Part model, mm, in its own coordinate system. Face numbers are marked on the shaded views. A direction names the side the tool comes from. Give positions to 0.01 mm unless a question says otherwise; leave off trailing zeros. Loops run counter-clockwise (first coordinate to the right, second up) from the corner with the lowest first, then second, coordinate; pieces in that order, holes last. Notation, with made-up numbers: (-12.5, 56.5) -> (20.5, 56.5) arc R21 ccw to (20.5, 94.5) -> close; hole circle Ø9 at (-4, 4.5). An arc over 180 degrees is marked (long way). Write item = value, one per line.
from build123d import *

# Parameters (mm, degrees)
F0_W      = 83.106392
F0_H      = 83.106392
F1_DEPTH  = 76.2
F2_T      = -2.54
F3_W      = 78.026392
F3_H      = 78.026392
F3_W_2    = 72.946392
F3_H_2    = 72.946392
F4_DEPTH  = 2.54
F8_DEPTH  = 2.54
F9_DEPTH  = 25.4
F11_DEPTH = 2.54
F12_DEPTH = 25.4


with BuildPart() as f1:
    # F0 (on Top) → F1 (new body)
    with BuildSketch(Plane.XY):
        Rectangle(F0_W, F0_H)
    extrude(amount=F1_DEPTH)

    # F2
    f2_openings = [f1.faces().sort_by_distance(p)[0] for p in [
        (0, 0, 76.2),
    ]]
    offset(amount=F2_T, openings=f2_openings)

    # F3 (on face) → F4 (join)
    with BuildSketch(Plane(origin=(0, 0, 0), x_dir=(1, 0, 0), z_dir=(0, 0, -1))):
        Rectangle(F3_W, F3_H)
        Rectangle(F3_W_2, F3_H_2, mode=Mode.SUBTRACT)
    extrude(amount=F4_DEPTH)

    # F5 (on face) → F8 (join)
    with BuildSketch(Plane(origin=(-41.553196, 0, 0), x_dir=(0, -1, 0), z_dir=(-1, 0, 0))):
        Polygon((-23.773196, 71.12), (-36.473196, 71.12), (-36.473196, 58.42), (-31.393196, 58.42), (-31.393196, 66.04), (-23.773196, 66.04), align=None)
        Polygon((36.473196, 58.42), (36.473196, 71.12), (23.773196, 71.12), (23.773196, 66.04), (31.393196, 66.04), (31.393196, 58.42), align=None)
        Polygon((36.473196, 17.78), (31.393196, 17.78), (31.393196, 10.16), (23.773196, 10.16), (23.773196, 5.08), (36.473196, 5.08), align=None)
        Polygon((-36.473196, 17.78), (-36.473196, 5.08), (-23.773196, 5.08), (-23.773196, 10.16), (-31.393196, 10.16), (-31.393196, 17.78), align=None)
    extrude(amount=F8_DEPTH)

    # F7 (on face) → F9 (cut)
    with BuildSketch(Plane.YZ.offset(41.553196)):
        Polygon((-23.773196, 71.12), (-36.473196, 71.12), (-36.473196, 58.42), (-31.393196, 58.42), (-31.393196, 66.04), (-23.773196, 66.04), align=None)
        Polygon((36.473196, 58.42), (36.473196, 71.12), (23.773196, 71.12), (23.773196, 66.04), (31.393196, 66.04), (31.393196, 58.42), align=None)
        Polygon((23.773196, 5.08), (36.473196, 5.08), (36.473196, 17.78), (31.393196, 17.78), (31.393196, 10.16), (23.773196, 10.16), align=None)
        Polygon((-36.473196, 17.78), (-36.473196, 5.08), (-23.773196, 5.08), (-23.773196, 10.16), (-31.393196, 10.16), (-31.393196, 17.78), align=None)
    extrude(amount=-F9_DEPTH, mode=Mode.SUBTRACT)

    # F10 (on face) → F11 (join)
    with BuildSketch(Plane(origin=(0, 41.553196, 0), x_dir=(-1, 0, 0), z_dir=(0, 1, 0))):
        Polygon((36.473196, 58.42), (36.473196, 71.12), (23.773196, 71.12), (23.773196, 66.04), (31.393196, 66.04), (31.393196, 58.42), align=None)
        Polygon((23.773196, 5.08), (36.473196, 5.08), (36.473196, 17.78), (31.393196, 17.78), (31.393196, 10.16), (23.773196, 10.16), align=None)
        Polygon((-36.473196, 17.78), (-36.473196, 5.08), (-23.773196, 5.08), (-23.773196, 10.16), (-31.393196, 10.16), (-31.393196, 17.78), align=None)
        Polygon((-23.773196, 71.12), (-36.473196, 71.12), (-36.473196, 58.42), (-31.393196, 58.42), (-31.393196, 66.04), (-23.773196, 66.04), align=None)
    extrude(amount=F11_DEPTH)

    # F6 (on face) → F12 (cut)
    with BuildSketch(Plane.XZ.offset(41.553196)):
        Polygon((-23.773196, 71.12), (-36.473196, 71.12), (-36.473196, 58.42), (-31.393196, 58.42), (-31.393196, 66.04), (-23.773196, 66.04), align=None)
        Polygon((-36.473196, 17.78), (-36.473196, 5.08), (-23.773196, 5.08), (-23.773196, 10.16), (-31.393196, 10.16), (-31.393196, 17.78), align=None)
        Polygon((23.773196, 5.08), (36.473196, 5.08), (36.473196, 17.78), (31.393196, 17.78), (31.393196, 10.16), (23.773196, 10.16), align=None)
        Polygon((36.473196, 58.42), (36.473196, 71.12), (23.773196, 71.12), (23.773196, 66.04), (31.393196, 66.04), (31.393196, 58.42), align=None)
    extrude(amount=-F12_DEPTH, mode=Mode.SUBTRACT)


solid = f1.part
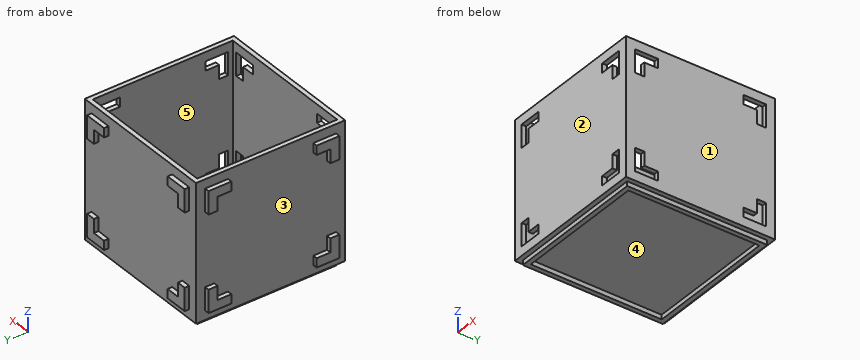
1) Drill centre lines: line 1 along X through (y, z) = (37, 14.5); line 2 along Z through (x, y) = (10, -3). Where is each one in solid material? Low to high. Write a range as [from, to].
Resolved:
line_1 = [-41.55, -39.01], [39.01, 41.55]
line_2 = [0, 2.54]
2) Which spindle directions (+Z, -Z, +X, -X, +Y, -Y) get a long thin tool onto all of the face, cutting with end or side? Do the marked faces 4 and 5. Say none if no direction does.
Resolved:
face_4 = -Z
face_5 = +Z
3) Pull direction Y, two halves, no side cores. Call the marked faces 1, 2 and 3: pulls with the +Y half, pulls with the -Y half, needs draft (parallel to the pull), parting line crosses it, or undercut.
Resolved:
face_1 = needs draft
face_2 = pulls with the -Y half
face_3 = undercut
4) Slice it at A-A, the plane x = -25.5. Count the separate pieces of the cut face and the enclosed holes in it, and give its area (3 significant figures).
Resolved:
separate_pieces = 3
enclosed_holes = 0
area = 598 mm²
5) Slice it at C-C, the plane z = 25. List the corners of the cut face in (x, y), and give its area (3 significant figures).
Resolved:
outline = (-41.55, -41.55) -> (41.55, -41.55) -> (41.55, 41.55) -> (-41.55, 41.55) -> close; hole (-39.01, -39.01) -> (39.01, -39.01) -> (39.01, 39.01) -> (-39.01, 39.01) -> close
area = 819 mm²
6) Drop flat-ended pins along their axis: P1, Ø10, axis at x = 12.5, y = 0.5, coming from the -Z side; P2, Ø0.8, axis at x = 30, y = 42, coming from the +Z side; P3, Ø1, axis at x = 13, z = 41, coming from the +Y side. Give the stop position or say it passes through.
Resolved:
P1 = 0
P2 = 71.12
P3 = 41.55
